For this review, take the finished solid that the model builds, in its own axes (mm). A direction names the side the tool comes from. Round coordinates to 2 decimals unless told otherwise and drop trailing zeros. Order: outer loops, then holes, each group sorted by start corner. A loop starts at its lowest first (then second) coordinate and runs counter-clockwise, first axis right, second up. Notation, with made-up numbers: M -33,24 L -12,24 A9 ccw -12,30 Z; hole C 42.5,86 d3. An arc over 180 degrees is marked long. Write item = value, one per line. Start each with the question number.
from build123d import *

# Parameters (mm, degrees)
BOSS_EXTRUDE1_DEPTH     = 31.85
CUT_EXTRUDE1_DEPTH      = 41.316226572
CUT_EXTRUDE1_DEPTH_BACK = 24.55
SHELL1_START            = -30.25
SHELL1_DEPTH            = 28.65
SHELL1_2_OUTLINE_W      = 35.35
SHELL1_2_OUTLINE_H      = 4.8
SHELL1_2_DEPTH          = 4.1
BOSS_EXTRUDE2_START     = -4.6
SKETCH3_R               = 1.5
SKETCH3_R_2             = 0.55
BOSS_EXTRUDE2_DEPTH     = 4.6
SKETCH4_W               = 32.15
SKETCH4_H               = 17.25
CUT_EXTRUDE2_DEPTH      = 1.95
SKETCH5_W               = 32.15
SKETCH5_H               = 4.65
CUT_EXTRUDE3_DEPTH      = 2.25
SKETCH6_R               = 2.45
BOSS_EXTRUDE3_DEPTH     = 1.85
SKETCH7_R               = 0.95
CUT_EXTRUDE4_DEPTH      = 1.65


# Read off the part's stored shape, not the designer's step: Shell1
with BuildPart() as part:
    # Sketch1 → Boss-Extrude1 (new body)
    with BuildSketch(Plane.XY):
        Polygon((23.875, 0), (23.875, 3), (20.2, 6.4), (-20.2, 6.4), (-23.875, 3), (-23.875, 0), align=None)
    extrude(amount=-BOSS_EXTRUDE1_DEPTH)

    # Sketch2 → Cut-Extrude1 (cut, two sides: drawn at the far end of the back side and taken through both)
    with BuildSketch(Plane.XY.offset(-CUT_EXTRUDE1_DEPTH_BACK)):
        Polygon((-16.075, -90.918786447), (-16.075, 0), (-16.075, 3.25), (16.075, 3.25), (16.075, 0), (16.075, -90.918786447), (16.075, -272.75635934), (-16.075, -272.75635934), align=None)
    extrude(amount=CUT_EXTRUDE1_DEPTH + CUT_EXTRUDE1_DEPTH_BACK, mode=Mode.SUBTRACT)

    # Shell1 outline → Shell1 (cut)
    with BuildSketch(Plane.XY.offset(SHELL1_START)):
        Polygon((22.275, 2.30054609), (19.573384377, 4.8), (17.675, 4.8), (17.675, 0), (22.275, 0), align=None)
        Polygon((-17.675, 0), (-17.675, 4.8), (-19.573384377, 4.8), (-22.275, 2.30054609), (-22.275, 0), align=None)
    extrude(amount=SHELL1_DEPTH, mode=Mode.SUBTRACT)

    # Shell1 2 outline → Shell1 2 (cut)
    with BuildSketch(Plane.XY.offset(SHELL1_START)):
        with Locations((0, 2.4)):
            Rectangle(SHELL1_2_OUTLINE_W, SHELL1_2_OUTLINE_H)
    extrude(amount=SHELL1_2_DEPTH, mode=Mode.SUBTRACT)

    # Sketch3 → Boss-Extrude2 (add)
    # profile 1 of 6: a face of its own
    with BuildSketch(Plane(origin=(0, 0.2, 0), x_dir=(-1, 0, 0), z_dir=(0, -1, 0)).offset(BOSS_EXTRUDE2_START)):
        with Locations(Location((19.975, 7.9625, 0), (0, 0, 90))):
            Circle(SKETCH3_R)
        with Locations(Location((19.975, 7.9625, 0), (0, 0, 90))):
            Circle(SKETCH3_R_2, mode=Mode.SUBTRACT)
    # profile 2 of 6: a face of its own
    with BuildSketch(Plane(origin=(0, 0.2, 0), x_dir=(-1, 0, 0), z_dir=(0, -1, 0)).offset(BOSS_EXTRUDE2_START)):
        with Locations(Location((19.975, 15.925, 0), (0, 0, 90))):
            Circle(SKETCH3_R)
        with Locations(Location((19.975, 15.925, 0), (0, 0, 90))):
            Circle(SKETCH3_R_2, mode=Mode.SUBTRACT)
    # profile 3 of 6: a face of its own
    with BuildSketch(Plane(origin=(0, 0.2, 0), x_dir=(-1, 0, 0), z_dir=(0, -1, 0)).offset(BOSS_EXTRUDE2_START)):
        with Locations(Location((19.975, 23.8875, 0), (0, 0, 90))):
            Circle(SKETCH3_R)
        with Locations(Location((19.975, 23.8875, 0), (0, 0, 90))):
            Circle(SKETCH3_R_2, mode=Mode.SUBTRACT)
    # profile 4 of 6: a face of its own
    with BuildSketch(Plane(origin=(0, 0.2, 0), x_dir=(-1, 0, 0), z_dir=(0, -1, 0)).offset(BOSS_EXTRUDE2_START)):
        with Locations(Location((-19.975, 23.8875, 0), (0, 0, 74.469949242))):
            Circle(SKETCH3_R)
        with Locations(Location((-19.975, 23.8875, 0), (0, 0, 43.095979253))):
            Circle(SKETCH3_R_2, mode=Mode.SUBTRACT)
    # profile 5 of 6: a face of its own
    with BuildSketch(Plane(origin=(0, 0.2, 0), x_dir=(-1, 0, 0), z_dir=(0, -1, 0)).offset(BOSS_EXTRUDE2_START)):
        with Locations(Location((-19.975, 15.925, 0), (0, 0, 74.469949242))):
            Circle(SKETCH3_R)
        with Locations(Location((-19.975, 15.925, 0), (0, 0, 43.095979253))):
            Circle(SKETCH3_R_2, mode=Mode.SUBTRACT)
    # profile 6 of 6: a face of its own
    with BuildSketch(Plane(origin=(0, 0.2, 0), x_dir=(-1, 0, 0), z_dir=(0, -1, 0)).offset(BOSS_EXTRUDE2_START)):
        with Locations(Location((-19.975, 7.9625, 0), (0, 0, 74.469949242))):
            Circle(SKETCH3_R)
        with Locations(Location((-19.975, 7.9625, 0), (0, 0, 43.095979253))):
            Circle(SKETCH3_R_2, mode=Mode.SUBTRACT)
    extrude(amount=BOSS_EXTRUDE2_DEPTH)

    # Sketch4 → Cut-Extrude2 (cut)
    with BuildSketch(Plane.XZ.offset(-3.25)):
        with Locations((0, -15.925)):
            Rectangle(SKETCH4_W, SKETCH4_H)
    extrude(amount=-CUT_EXTRUDE2_DEPTH, mode=Mode.SUBTRACT)

    # Sketch5 → Cut-Extrude3 (cut)
    with BuildSketch(Plane.XZ.offset(-3.25)):
        with Locations((0, -3.825)):
            Rectangle(SKETCH5_W, SKETCH5_H)
    extrude(amount=-CUT_EXTRUDE3_DEPTH, mode=Mode.SUBTRACT)

    # Sketch6 → Boss-Extrude3 (add)
    with BuildSketch(Plane(origin=(0, 6.4, 0), x_dir=(1, 0, 0), z_dir=(0, 1, 0))):
        with Locations(Location((-3.98, 3.98, 0), (0, 0, 270))):
            Circle(SKETCH6_R)
        with Locations(Location((3.98, 3.98, 0), (0, 0, 270))):
            Circle(SKETCH6_R)
        with Locations(Location((-11.94, 3.98, 0), (0, 0, 270))):
            Circle(SKETCH6_R)
        with Locations(Location((11.94, 3.98, 0), (0, 0, 270))):
            Circle(SKETCH6_R)
    extrude(amount=BOSS_EXTRUDE3_DEPTH)

    # Sketch7 → Cut-Extrude4 (cut)
    with BuildSketch(Plane.XZ.offset(-5.5)):
        with Locations(Location((-11.94, -3.98, 0), (0, 0, 270))):
            Circle(SKETCH7_R)
        with Locations(Location((-3.98, -3.98, 0), (0, 0, 270))):
            Circle(SKETCH7_R)
        with Locations(Location((3.98, -3.98, 0), (0, 0, 270))):
            Circle(SKETCH7_R)
        with Locations(Location((11.94, -3.98, 0), (0, 0, 270))):
            Circle(SKETCH7_R)
    extrude(amount=-CUT_EXTRUDE4_DEPTH, mode=Mode.SUBTRACT)


solid = part.part
(1) We need section A-A, the plane z = -20.5. Write out the cut boundary in (x, y) (3 decimals), then the cut area to 3 significant figures.
(2) For faces 4 (the flat face through (-22.012, 4.724, -15.702)), 5 (the flat face through (-20, 2, -1.6)), 6 (the cylindrical face through (14.006, 7.312, -2.663)), list the 3-axis set-ups (+Z, -Z, +X, -X, +Y, -Y) from which the entire face can be reached by the end or side of a thin tool; tool diameter is ignored.
(3) For line 1 along X through (y, z) = (2.25, -5.5) (3 decimals); line 2 along Z through (x, y) = (-12, 6.25); line 3 along Z through (x, y) = (-14, 2.5), list the stretches that pass through material, from the lowest coordinate up.
(4) Draft analysis for pull direction Z (two halves, no side actions). For faces 1 (the flat face through (0, 4, 0)), 2 (the flat face through (-20.04, 4.37, -23.9)), 3 (the flat face through (-12, 8.25, -4)), state which applies: released by +Z, released by -Z, zero draft, split by the parting line, or undercut.
(5) Insertion check: pin 1 (16 mm diameter, centred on x = -1.5, z = -21, fed in from +Y); pin 2 (1.1 mm diameter, centred on x = 3.98, z = -3.98, fed in from -Y); pin 3 (1.5 mm diameter, centred on x = -11.5, z = -4, fed in from -Y). Each pin has a flat end and moves straight along its axis. Give the tip position at first contact, or say it passes through.
(6) We need section C-C, the plane x = 8. Write out the cut boundary in (y, z).
(7) We need section B-B, the plane x = -11.94. Write out the cut boundary in (y, z).
Values:
q1.outline = M -23.875,0 L -22.275,0 L -22.275,2.301 L -19.573,4.8 L -17.675,4.8 L -17.675,0 L -16.075,0 L -16.075,5.2 L 16.075,5.2 L 16.075,0 L 17.675,0 L 17.675,4.8 L 19.573,4.8 L 22.275,2.301 L 22.275,0 L 23.875,0 L 23.875,3 L 20.2,6.4 L -20.2,6.4 L -23.875,3 Z
q1.area = 88.5 mm²
q2.face_4 = +Z, -Z, -X, +Y
q2.face_5 = -Y
q2.face_6 = +Y
q3.line_1 = -23.875 to -22.275, -17.675 to -16.075, 16.075 to 17.675, 22.275 to 23.875
q3.line_2 = -31.85 to -4.93, -3.03 to 0
q3.line_3 = -31.85 to -30.25, -26.15 to -24.55
q4.face_1 = released by +Z
q4.face_2 = undercut
q4.face_3 = zero draft
q5.pin_1 = 6.4
q5.pin_2 = 7.15
q5.pin_3 = 5.5
q6.outline = M 0,-31.85 L 6.4,-31.85 L 6.4,0 L 3.25,0 L 3.25,-1.5 L 5.5,-1.5 L 5.5,-6.15 L 3.25,-6.15 L 3.25,-7.3 L 5.2,-7.3 L 5.2,-24.55 L 0,-24.55 L 0,-26.15 L 4.8,-26.15 L 4.8,-30.25 L 0,-30.25 Z
q7.outline = M 0,-31.85 L 6.4,-31.85 L 6.4,-6.43 L 8.25,-6.43 L 8.25,-1.53 L 6.4,-1.53 L 6.4,0 L 3.25,0 L 3.25,-1.5 L 5.5,-1.5 L 5.5,-3.03 L 7.15,-3.03 L 7.15,-4.93 L 5.5,-4.93 L 5.5,-6.15 L 3.25,-6.15 L 3.25,-7.3 L 5.2,-7.3 L 5.2,-24.55 L 0,-24.55 L 0,-26.15 L 4.8,-26.15 L 4.8,-30.25 L 0,-30.25 Z
